from build123d import *

# Parameters (mm, degrees)
PLAT_W                      = 100
PLAT_H                      = 10
EL_MENT_M_CANO_SOUD_1_DEPTH = 150
D_GAGEMENT_M121_D           = 13


with BuildPart() as part:
    # plat → Elément mécano-soudé1 (new body)
    with BuildSketch(Plane.YZ):
        Rectangle(PLAT_W, PLAT_H)
    extrude(amount=EL_MENT_M_CANO_SOUD_1_DEPTH)

    # Dégagement M121 (through all)
    with Locations(Plane.XY.offset(5)):
        with Locations((13.5, 36.5), (136.5, 36.5), (136.5, -36.5), (13.5, -36.5)):
            Hole(D_GAGEMENT_M121_D / 2)


solid = part.part
Model file for the job. Use its own axes, mm. Give positions to 0.01 mm unless a question says otherwise; leave off trailing zeros. Loops run counter-clockwise (first coordinate to the right, second up) from the corner with the lowest first, then second, coordinate; pieces in that order, holes last.
1) Saw through at C-C (z = 0.25). Write the cut outline in (x, y).
2) Pull direction X, two halves, no side cores. Call faces 1 (the flat face through (0, -1, 0)), 2 (the cylindrical face through (142.994, -36.214, -0.07)), 3 (the flat face through (74, 50, 0)): +X half, -X half, draft (parallel to the pull), parting line (faces both ways), or undercut.
3) Saw through at A-A (x = 136.5). Write the cut outline in (y, z), plus the area to 3 significant figures.
4) Saw through at B-B (y = -39). Write the cut outline in (x, z), plus the area to 3 significant figures.
5) Wall check: line 1 (Y direction, x = 13.5, z = -0.25); line 2 (Y direction, x = 16, z = -3.5); line 3 (X direction, y = 30.5, z = -2.25). Give the ranges that are in metal, low to high.
Answer block:
1. outline: (0, -50) - (150, -50) - (150, 50) - (0, 50) - close; hole circle Ø13 at (13.5, -36.5); hole circle Ø13 at (13.5, 36.5); hole circle Ø13 at (136.5, -36.5); hole circle Ø13 at (136.5, 36.5)
2. face 1: -X half
2. face 2: undercut
2. face 3: draft
3. outline: (-50, -5) - (-43, -5) - (-43, 5) - (-50, 5) - close; (-30, -5) - (30, -5) - (30, 5) - (-30, 5) - close; (43, -5) - (50, -5) - (50, 5) - (43, 5) - close
3. area: 740 mm2
4. outline: (0, -5) - (7.5, -5) - (7.5, 5) - (0, 5) - close; (19.5, -5) - (130.5, -5) - (130.5, 5) - (19.5, 5) - close; (142.5, -5) - (150, -5) - (150, 5) - (142.5, 5) - close
4. area: 1,260 mm2
5. line 1: y = -50 to -43, -30 to 30, 43 to 50
5. line 2: y = -50 to -42.5, -30.5 to 30.5, 42.5 to 50
5. line 3: x = 0 to 11, 16 to 134, 139 to 150
